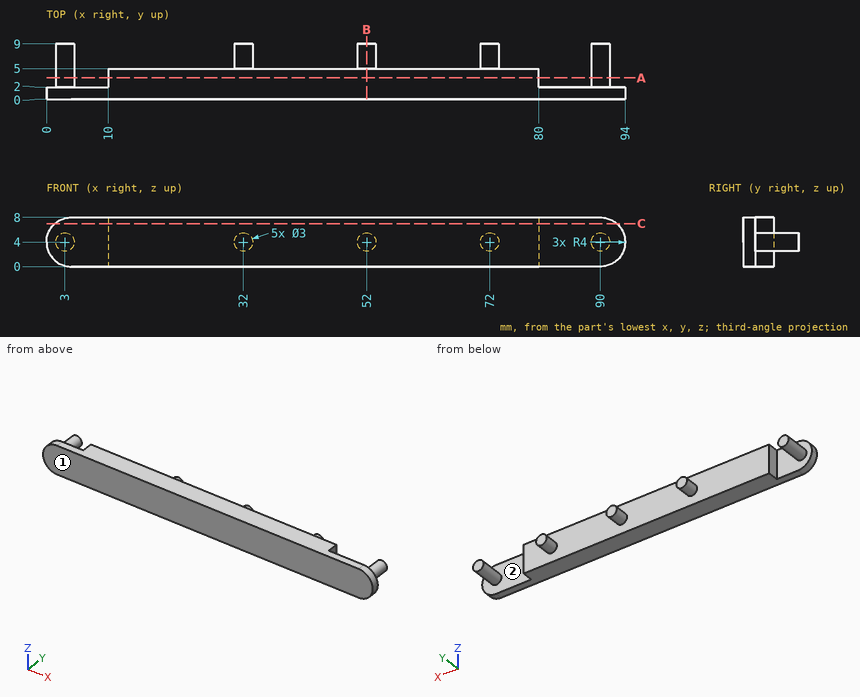
Can you work these out from the drawing? Everything is in mm from the part's minimum corner. Round coordinates to 2 decimals unless told otherwise and drop trailing zeros. Order: outer loops, then holes, each group sorted by start corner. A loop starts at its lowest first (then second) coordinate and runs counter-clockwise, first axis right, second up. Notation, with made-up numbers: M -2,-26 L 8,-26 A17 cw 8,-13 Z; hole C 72.5,-17 d7. An arc over 180 degrees is marked long. Answer as CSV lines item,"result".
Item 1: Imagine slicing it at C-C on z = 7. List the corners of the cut face in (x, y) for me, and give its area (3 significant figures).
From the geometry:
outline,"M 1.35,0 L 92.65,0 L 92.65,2 L 80,2 L 80,5 L 10,5 L 10,2 L 1.35,2 Z"
area,"393 mm2"
Item 2: For pin 1 (1.5 mm diameter, centred on y = 3.5, z = 4.5, fed in from -X); pin 2 (3.5 mm diameter, centred on y = 3.5, z = 2.5, fed in from +X) (3 decimals); pin 3 (4 mm diameter, centred on x = 48, y = 1.5, fed in from -Z); pin 4 (2.5 mm diameter, centred on x = 84.5, z = 2, fed in from +Y), each with a flat end and sliding along its axis, tell me the tip position at first contact or that it passes through.
From the geometry:
pin 1,"x = 1.5"
pin 2,"x = 93.955"
pin 3,"z = 0"
pin 4,"y = 2"
Item 3: Imagine slicing it at A-A on y = 3.5. List the corners of the cut face in (x, z) for me.
From the geometry:
outline,"C 3,4 d3; M 10,0 L 80,0 L 80,8 L 10,8 Z; C 90,4 d3"
Item 4: Imagine slicing it at B-B on x = 52. List the corners of the cut face in (y, z) for me, and give its area (3 significant figures).
From the geometry:
outline,"M 0,0 L 5,0 L 5,2.5 L 9,2.5 L 9,5.5 L 5,5.5 L 5,8 L 0,8 Z"
area,"52.0 mm2"
Item 5: We'd pull the mould along X, two halves only. Please class the marked faces 1 and 2: +X half, -X half, draft (parallel to the pull), parting line (faces both ways), or undercut.
From the geometry:
face 1,"draft"
face 2,"undercut"
Item 6: Please list where these lines run through material, in increasing order: L1, parallel to X at y = 2.75, z = 5.25; L2, parallel to X at y = 2.5, z = 2.25; L3, parallel to Y at x = 61, z = 5.75. Write a range as [from, to].
From the geometry:
L1,"[2.17, 3.83], [10, 80], [89.17, 90.83]"
L2,"[10, 80]"
L3,"[0, 5]"
